from build123d import *

# Parameters (mm, degrees)
BASE_DEPTH                 = 12
SCREWS_ZIP_TIE_HOLES_REACH = 30.539
SKETCH2_R                  = 1.4
SKETCH2_W                  = 5
SKETCH2_H                  = 3
F_1MM_EDGE_FILLETS_R       = 1


with BuildPart() as part:
    # Sketch1 → Base (new body)
    with BuildSketch(Plane(origin=(0, 0, 0), x_dir=(1, 0, 0), z_dir=(0, 1, 0))):
        with BuildLine():
            Line((4.5, 25.5), (4.5, 15.5))
            ThreePointArc((4.5, 15.5), (3.297918472, 15.002081528), (2.8, 13.8))
            Line((2.8, 13.8), (2.8, 11.2))
            ThreePointArc((2.8, 11.2), (3.297918472, 9.997918472), (4.5, 9.5))
            Line((4.5, 9.5), (4.5, -9.5))
            ThreePointArc((4.5, -9.5), (3.297918472, -9.997918472), (2.8, -11.2))
            Line((2.8, -11.2), (2.8, -13.8))
            ThreePointArc((2.8, -13.8), (3.297918472, -15.002081528), (4.5, -15.5))
            Line((4.5, -15.5), (4.5, -25.5))
            Line((4.5, -25.5), (0, -25.5))
            Line((0, -25.5), (0, 25.5))
            Line((0, 25.5), (4.5, 25.5))
        make_face()
    extrude(amount=BASE_DEPTH)

    # Sketch2 → Screws _ Zip Tie Holes (cut, up to next)
    with BuildSketch(Plane(origin=(4.5, 0, 0), x_dir=(0, 0, -1), z_dir=(1, 0, 0)), mode=Mode.PRIVATE) as screws_zip_tie_holes_sk1:
        with Locations((-4.5, 6)):
            Circle(SKETCH2_R)
    screws_zip_tie_holes_tool1 = extrude(screws_zip_tie_holes_sk1.sketch, amount=-SCREWS_ZIP_TIE_HOLES_REACH, mode=Mode.PRIVATE) & part.part
    # Sketch2 → Screws _ Zip Tie Holes (cut, up to next)
    with BuildSketch(Plane(origin=(4.5, 0, 0), x_dir=(0, 0, -1), z_dir=(1, 0, 0)), mode=Mode.PRIVATE) as screws_zip_tie_holes_sk2:
        with Locations((4.5, 6)):
            Circle(SKETCH2_R)
    screws_zip_tie_holes_tool2 = extrude(screws_zip_tie_holes_sk2.sketch, amount=-SCREWS_ZIP_TIE_HOLES_REACH, mode=Mode.PRIVATE) & part.part
    # Sketch2 → Screws _ Zip Tie Holes (cut, up to next)
    with BuildSketch(Plane(origin=(4.5, 0, 0), x_dir=(0, 0, -1), z_dir=(1, 0, 0)), mode=Mode.PRIVATE) as screws_zip_tie_holes_sk3:
        with Locations((20.5, 6)):
            Rectangle(SKETCH2_W, SKETCH2_H)
    screws_zip_tie_holes_tool3 = extrude(screws_zip_tie_holes_sk3.sketch, amount=-SCREWS_ZIP_TIE_HOLES_REACH, mode=Mode.PRIVATE) & part.part
    # Sketch2 → Screws _ Zip Tie Holes (cut, up to next)
    with BuildSketch(Plane(origin=(4.5, 0, 0), x_dir=(0, 0, -1), z_dir=(1, 0, 0)), mode=Mode.PRIVATE) as screws_zip_tie_holes_sk4:
        with Locations((-20.5, 6)):
            Rectangle(SKETCH2_W, SKETCH2_H)
    screws_zip_tie_holes_tool4 = extrude(screws_zip_tie_holes_sk4.sketch, amount=-SCREWS_ZIP_TIE_HOLES_REACH, mode=Mode.PRIVATE) & part.part
    add(screws_zip_tie_holes_tool1.solids().sort_by_distance((4.5, 6, 4.5))[0], mode=Mode.SUBTRACT)
    add(screws_zip_tie_holes_tool2.solids().sort_by_distance((4.5, 6, -4.5))[0], mode=Mode.SUBTRACT)
    add(screws_zip_tie_holes_tool3.solids().sort_by_distance((4.5, 6, -20.5))[0], mode=Mode.SUBTRACT)
    add(screws_zip_tie_holes_tool4.solids().sort_by_distance((4.5, 6, 20.5))[0], mode=Mode.SUBTRACT)

    # 1mm Edge Fillets
    f_1mm_edge_fillets_edges = [part.edges().sort_by_distance(p)[0] for p in [
        (2.25, 0, -25.5),
        (2.25, 0, 25.5),
        (0, 0, 0),
        (0, 6, -25.5),
        (0, 6, 25.5),
        (2.25, 12, -25.5),
        (0, 12, 0),
        (2.25, 12, 25.5),
    ]]
    fillet(f_1mm_edge_fillets_edges, radius=F_1MM_EDGE_FILLETS_R)


solid = part.part
Build history of the part. All positions in model axes, mm. A direction names the side the tool comes from. Give positions to 0.01 mm unless a question says otherwise; leave off trailing zeros. Loops run counter-clockwise (first coordinate to the right, second up) from the corner with the lowest first, then second, coordinate; pieces in that order, holes last. Notation, with made-up numbers: (34.25, 25) - (74.25, 25) arc R16 cw to (74.25, 55) - close; hole circle Ø7 at (-18, 76.5). An arc over 180 degrees is marked (long way). Write item = value, one per line. Start each with the question number.
1) Band-saw the part on A-A on z = 19.5. Give the cut face in (x, y).
2) Probe probe 1 along Y at (x, z) = (1.95, -4.5); probe 2 along Z at (x, y) = (3.45, 1.25); probe 3 along Y at (x, z) = (0.95, -2.5). List the from-to ranges inside material, lowest first. Write a range as from..to.
3) Band-saw the part on D-D on y = 6.75. Count the separate pieces of the cut face and the enclosed holes in it, plus the area to 3 significant figures.
4) Band-saw the part on C-C on y = 3.75. Give the cut face in (x, z), plus the area to 3 significant figures.
5) Tool access for faces 4 (the cylindrical face through (3.285, 5.916, -10.011)), 5 (the flat face through (4.5, 3, -21)), 6 (the flat face through (2, 6, 23)): list every direction of +Z, -Z, +X, -X, +Y, -Y with a clear straight run to the whole face (end or side of a thin tool).
6) Band-saw the part on B-B on x = 3.3. Give the cut face in (y, z), plus the area to 3 significant figures.
7) Pull direction Z, two halves, no side cores. Call faces 1 (the cylindrical face through (2.774, 11.699, -25.215)), 2 (the flat face through (2, 6, 18)), 3 (the cylindrical face through (0.301, 0.285, -0.343)): +Z half, -Z half, draft (parallel to the pull), parting line (faces both ways), or undercut.
8) Drop flat-ended pins along their axis: pin 1 Ø2 at (y, z) = (7, 12) entering from +X; pin 2 Ø2 at (y, z) = (6, 4.5) entering from +X. Give the stop position or say it passes through.
Final values:
q1.outline = (0, 1) arc R1 ccw to (1, 0) - (4.5, 0) - (4.5, 4.5) - (0, 4.5) - close; (0, 7.5) - (4.5, 7.5) - (4.5, 12) - (1, 12) arc R1 ccw to (0, 11) - close
q2.probe_1 = 0..4.6, 7.4..12
q2.probe_2 = -25.5..-15.14, -9.86..9.86, 15.14..25.5
q2.probe_3 = 0..12
q3.separate_pieces = 5
q3.enclosed_holes = 0
q3.area = 145 mm²
q4.outline = (0, -24.5) arc R1 ccw to (1, -25.5) - (4.5, -25.5) - (4.5, -15.5) arc R1.7 cw to (2.8, -13.8) - (2.8, -11.2) arc R1.7 cw to (4.5, -9.5) - (4.5, 9.5) arc R1.7 cw to (2.8, 11.2) - (2.8, 13.8) arc R1.7 cw to (4.5, 15.5) - (4.5, 25.5) - (1, 25.5) arc R1 ccw to (0, 24.5) - close
q4.area = 211 mm²
q5.face_4 = +X, +Y, -Y
q5.face_5 = +Z, -Z, +X, +Y, -Y
q5.face_6 = +X, -X
q6.outline = (0, -24.5) arc R1 ccw to (1, -25.5) - (11, -25.5) arc R1 ccw to (12, -24.5) - (12, -15) - (0, -15) - close; (0, -10) - (12, -10) - (12, 10) - (0, 10) - close; (0, 15) - (12, 15) - (12, 24.5) arc R1 ccw to (11, 25.5) - (1, 25.5) arc R1 ccw to (0, 24.5) - close; hole (4.5, -23) - (7.5, -23) - (7.5, -18) - (4.5, -18) - close; hole (4.5, 18) - (7.5, 18) - (7.5, 23) - (4.5, 23) - close; hole circle Ø2.8 at (6, -4.5); hole circle Ø2.8 at (6, 4.5)
q6.area = 449 mm²
q7.face_1 = -Z half
q7.face_2 = undercut
q7.face_3 = draft
q8.pin_1 = 2.81
q8.pin_2 = through
